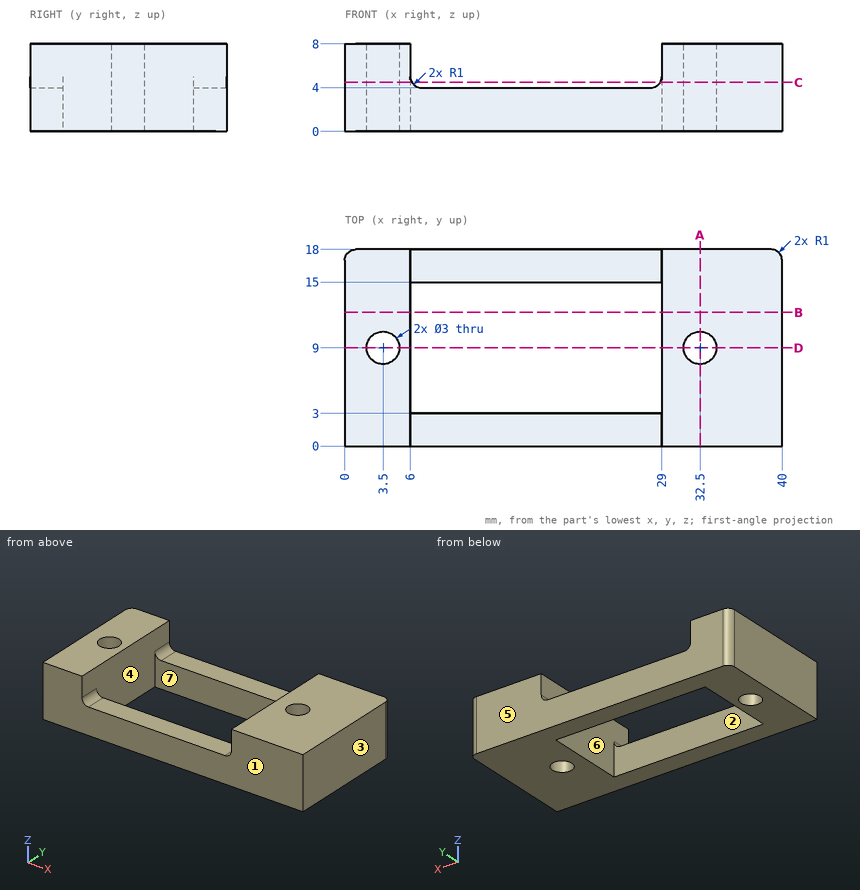
Study the drawing (mm; zero at the part's minimum x, y, z) and answer. A direction names the side the tool comes from. Give positions to 0.01 mm unless a question says otherwise; leave off trailing zeros. Write each loop counter-clockwise with the first axis right and the second up, starting at its lowest first coordinate (ties: lowest second). Pieces come first, ordered by that corner, then holes. Notation, with made-up numbers: (56.25, 32.25) -> (70.25, 32.25) arc R27 cw to (70.25, 57.25) -> close; hole circle Ø1 at (60, 13.25). An arc over 180 degrees is marked (long way). Answer as a JSON object with one key per item and string values. Group by question number.
1) Find section C-C (z = 4.5). Write down the section's boundary in (x, y).
2) Find section A-A (x = 32.5). Write down the section's boundary in (y, z).
3) The mould has two halves that part along X. Classify the marked faces 1, 2, 3 and 4: +X half, -X half, draft (parallel to the pull), parting line (faces both ways), or undercut.
4) A tool of negligible diameter and unlimited length cuts with its end or side. For the marked faces 5, 6 and 7, from which of +Z, -Z, +X, -X, +Y, -Y can it reach the whole face along a straight path? Write none if from no direction.
5) Consider L1, parallel to X at y = 9, z = 4.75; L2, parallel to Y at x = 14, z = 1; L3, parallel to Y at x = 32.5, z = 4.75. Determine where each line is inside the solid, lowest interval first. Write a range as from..to.
6) Find section B-B (y = 12.25). Write down the section's boundary in (x, z).
7) Find section D-D (y = 9). Write down the section's boundary in (x, z).
8) This flat-tipped pin is pushed along its axis until it touches: P1, Ø0.9, axis at x = 15, y = 1.5, coming from the +Z side. Where does it stop, or does it pass through?
Values follow:
{
 "1": {"outline": "(0, 0) -> (6.13, 0) -> (6.13, 3) -> (6, 3) -> (6, 15) -> (6.13, 15) -> (6.13, 18) -> (1, 18) arc R1 ccw to (0, 17) -> close; (28.87, 0) -> (40, 0) -> (40, 17) arc R1 ccw to (39, 18) -> (28.87, 18) -> (28.87, 15) -> (29, 15) -> (29, 3) -> (28.87, 3) -> close; hole circle Ø3 at (3.5, 9); hole circle Ø3 at (32.5, 9)"},
 "2": {"outline": "(0, 0) -> (7.5, 0) -> (7.5, 8) -> (0, 8) -> close; (10.5, 0) -> (18, 0) -> (18, 8) -> (10.5, 8) -> close"},
 "3": {"face 1": "draft", "face 2": "undercut", "face 3": "+X half", "face 4": "undercut"},
 "4": {"face 5": "+Z, -Z, +X, -X, +Y", "face 6": "+Z", "face 7": "+Z, -Z"},
 "5": {"L1": "x = 0..2, 5..6, 29..31, 34..40", "L2": "y = 0..3, 15..18", "L3": "y = 0..7.5, 10.5..18"},
 "6": {"outline": "(0, 0) -> (6, 0) -> (6, 8) -> (0, 8) -> close; (29, 0) -> (40, 0) -> (40, 8) -> (29, 8) -> close"},
 "7": {"outline": "(0, 0) -> (2, 0) -> (2, 8) -> (0, 8) -> close; (5, 0) -> (6, 0) -> (6, 8) -> (5, 8) -> close; (29, 0) -> (31, 0) -> (31, 8) -> (29, 8) -> close; (34, 0) -> (40, 0) -> (40, 8) -> (34, 8) -> close"},
 "8": {"P1": "stops at z = 4"}
}
